Part model, mm, in its own coordinate system. Face numbers are marked on the shaded views. A direction names the side the tool comes from. Give positions to 0.01 mm unless a question says otherwise; leave off trailing zeros. Write each loop counter-clockwise with the first axis right and the second up, starting at its lowest first coordinate (ties: lowest second). Pieces come first, ordered by that corner, then holes. Notation, with made-up numbers: M 56,20 L 99,20 A29 cw 99,52 Z; hole C 12,-2 d10. An arc over 180 degrees is marked long. Answer as CSV lines item,"result". Start each with the question number.
1) Wall check: line 1 along Y through (x, z) = (-5, 5.5); line 2 along Y through (x, z) = (10.75, -1); line 3 along X through (y, z) = (-16, -5.5). Give the ranges that are in metal, low to high. Write a range as from..to.
2) Slice it at A-A, the plane x = 0. Give the cut face in (y, z), plus the area to 3 significant figures.
3) Slice it at C-C, the plane y = -4. Give the cut face in (x, z), plus the area to 3 significant figures.
4) Pin check, flat tips, straight feed: pin 1 Ø1.9 at (x, y) = (0, -30) entering from +Z; pin 2 Ø5 at (x, z) = (3.5, -1.5) entering from -Y; pin 3 Ø2.5 at (y, z) = (-31, -0.5) entering from +X; pin 4 Ø3 at (x, y) = (-2.5, -4) entering from +Z. Stop position of each tip, or through.
5) Slice it at D-D, the plane x = 7.5. Give the cut face in (y, z), plus the area to 3 significant figures.
6) Tool access for the marked faces 1, 2 and 3: list every direction of +Z, -Z, +X, -X, +Y, -Y with a clear straight run to the whole face (end or side of a thin tool).
7) Slice it at B-B, the plane z = -1.5. Give the cut face in (x, y).
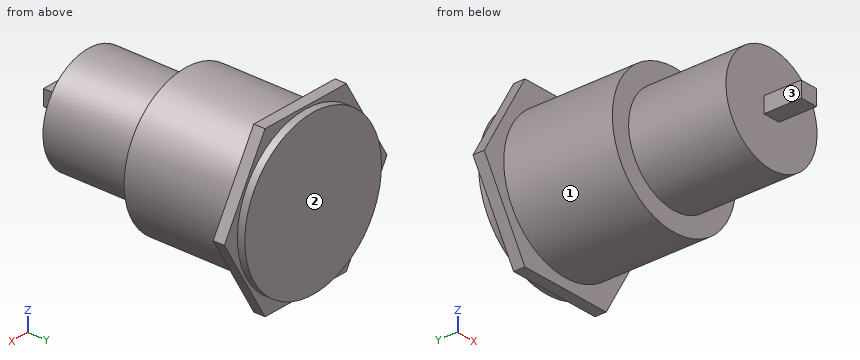
```python
from build123d import *

# Parameters (mm, degrees)
SKETCH1_R           = 9.5
BOSS_EXTRUDE1_DEPTH = 14.5
SKETCH2_R           = 7
BOSS_EXTRUDE2_DEPTH = 13
BOSS_EXTRUDE3_DEPTH = 1.5
SKETCH4_R           = 10.5
BOSS_EXTRUDE4_DEPTH = 1
SKETCH5_W           = 2.336545246
SKETCH5_H           = 2.080922042
BOSS_EXTRUDE5_DEPTH = 5


with BuildPart() as part:
    # Sketch1 → Boss-Extrude1 (new body)
    with BuildSketch(Plane(origin=(0, 0, 0), x_dir=(1, 0, 0), z_dir=(0, 1, 0))):
        with Locations(Location((0, 0, 0), (0, 0, 270))):
            Circle(SKETCH1_R)
    extrude(amount=-BOSS_EXTRUDE1_DEPTH)

    # Sketch2 → Boss-Extrude2 (add)
    with BuildSketch(Plane.XZ.offset(14.5)):
        with Locations(Location((0, 0, 0), (0, 0, 270))):
            Circle(SKETCH2_R)
    extrude(amount=BOSS_EXTRUDE2_DEPTH)

    # Sketch3 → Boss-Extrude3 (add)
    with BuildSketch(Plane(origin=(0, 0, 0), x_dir=(1, 0, 0), z_dir=(0, 1, 0))):
        Polygon((12.5, 0), (6.25, 10.825317547), (-6.25, 10.825317547), (-12.5, 0), (-6.25, -10.825317547), (6.25, -10.825317547), align=None)
    extrude(amount=BOSS_EXTRUDE3_DEPTH)

    # Sketch4 → Boss-Extrude4 (add)
    with BuildSketch(Plane(origin=(0, 1.5, 0), x_dir=(1, 0, 0), z_dir=(0, 1, 0))):
        with Locations(Location((0, 0, 0), (0, 0, 270))):
            Circle(SKETCH4_R)
    extrude(amount=BOSS_EXTRUDE4_DEPTH)

    # Sketch5 → Boss-Extrude5 (add)
    with BuildSketch(Plane.XZ.offset(27.5)):
        Rectangle(SKETCH5_W, SKETCH5_H)
    extrude(amount=BOSS_EXTRUDE5_DEPTH)


solid = part.part
```
Found:
1,line 1,"-14.5..2.5"
1,line 2,"0..1.5"
1,line 3,"-4.33..4.33"
2,outline,"M -32.5,-1.04 L -27.5,-1.04 L -27.5,-7 L -14.5,-7 L -14.5,-9.5 L 0,-9.5 L 0,-10.83 L 1.5,-10.83 L 1.5,-10.5 L 2.5,-10.5 L 2.5,10.5 L 1.5,10.5 L 1.5,10.83 L 0,10.83 L 0,9.5 L -14.5,9.5 L -14.5,7 L -27.5,7 L -27.5,1.04 L -32.5,1.04 Z"
2,area,"521 mm²"
3,outline,"C 0,0 d19"
3,area,"284 mm²"
4,pin 1,"z = 1.04"
4,pin 2,"y = -32.5"
4,pin 3,"x = 1.17"
4,pin 4,"z = 9.45"
5,outline,"M -14.5,-5.83 L 0,-5.83 L 0,-8.66 L 1.5,-8.66 L 1.5,-7.35 L 2.5,-7.35 L 2.5,7.35 L 1.5,7.35 L 1.5,8.66 L 0,8.66 L 0,5.83 L -14.5,5.83 Z"
5,area,"210 mm²"
6,face 1,"-Y"
6,face 2,"+Z, -Z, +X, -X, +Y"
6,face 3,"+Z, -Z, -X, -Y"
7,outline,"M -11.63,0 L -9.38,0 L -9.38,-14.5 L -6.84,-14.5 L -6.84,-27.5 L 6.84,-27.5 L 6.84,-14.5 L 9.38,-14.5 L 9.38,0 L 11.63,0 L 11.63,1.5 L 10.39,1.5 L 10.39,2.5 L -10.39,2.5 L -10.39,1.5 L -11.63,1.5 Z"
